```python
from build123d import *

# Parameters (mm, degrees)
SKETCH1_W               = 50.8
SKETCH1_H               = 304.8
BOSS_EXTRUDE1_DEPTH     = 3.175
CUT_EXTRUDE1_DEPTH      = 155.53478775
CUT_EXTRUDE1_DEPTH_BACK = 155.53478775
SKETCH2_R               = 3.175


with BuildPart() as part:
    # Sketch1 → Boss-Extrude1 (new, symmetric)
    with BuildSketch(Plane.XY):
        Rectangle(SKETCH1_W, SKETCH1_H)
    extrude(amount=BOSS_EXTRUDE1_DEPTH, both=True)

    # Sketch2 → Cut-Extrude1 (cut, two sides: drawn at the far end of the back side and taken through both)
    with BuildSketch(Plane.XY.offset(-CUT_EXTRUDE1_DEPTH_BACK)):
        with Locations((-12.7, 127)):
            Circle(SKETCH2_R)
        with Locations((12.7, 127)):
            Circle(SKETCH2_R)
        with Locations((12.7, 101.6)):
            Circle(SKETCH2_R)
        with Locations((12.7, 76.2)):
            Circle(SKETCH2_R)
        with Locations((12.7, 50.8)):
            Circle(SKETCH2_R)
        with Locations((12.7, 25.4)):
            Circle(SKETCH2_R)
        with Locations((12.7, 0)):
            Circle(SKETCH2_R)
        with Locations((12.7, -25.4)):
            Circle(SKETCH2_R)
        with Locations((12.7, -50.8)):
            Circle(SKETCH2_R)
        with Locations((12.7, -76.2)):
            Circle(SKETCH2_R)
        with Locations((12.7, -101.6)):
            Circle(SKETCH2_R)
        with Locations((-12.7, 101.6)):
            Circle(SKETCH2_R)
        with Locations((-12.7, 76.2)):
            Circle(SKETCH2_R)
        with Locations((-12.7, 50.8)):
            Circle(SKETCH2_R)
        with Locations((-12.7, 25.4)):
            Circle(SKETCH2_R)
        with Locations((-12.7, 0)):
            Circle(SKETCH2_R)
        with Locations((-12.7, -25.4)):
            Circle(SKETCH2_R)
        with Locations((-12.7, -50.8)):
            Circle(SKETCH2_R)
        with Locations((-12.7, -76.2)):
            Circle(SKETCH2_R)
        with Locations((-12.7, -101.6)):
            Circle(SKETCH2_R)
        with Locations((-12.7, -127)):
            Circle(SKETCH2_R)
        with Locations((12.7, -127)):
            Circle(SKETCH2_R)
    extrude(amount=CUT_EXTRUDE1_DEPTH + CUT_EXTRUDE1_DEPTH_BACK, mode=Mode.SUBTRACT)


solid = part.part
```
Geometry check sheet. Reference: the model listing, model coordinates, mm. Give positions to 0.01 mm unless a question says otherwise; leave off trailing zeros. Order: outer loops, then holes, each group sorted by start corner. A loop starts at its lowest first (then second) coordinate and runs counter-clockwise, first axis right, second up.
1. Release check for a two-part mould opening along X. For faces 1 (the face through (0, 152.4, 0)), 2 (the face through (-25.4, -2, 0)), 3 (the face through (12.29, -123.85, -0.04)) record: pulls with the +X half, pulls with the -X half, needs draft (parallel to the pull), parting line crosses it, or undercut.
2. Section check B-B, the plane z = 0.75. Give the number of separate pieces and of enclosed holes in the cut face, and give its area (3 significant figures).
3. Thickness scan on L1, parallel to X at y = 127, z = 1 (3 decimals); L2, parallel to X at y = 99, z = -1.75. Record the ranges inside material, lowest first.
4. Section check A-A, the plane y = 101.6. Enter the section's corners in (x, z) (3 decimals).
Values follow:
1. face 1: needs draft
1. face 2: pulls with the -X half
1. face 3: undercut
2. separate pieces: 1
2. enclosed holes: 22
2. area: 14,800 mm2
3. L1: x = -25.4 to -15.875, -9.525 to 9.525, 15.875 to 25.4
3. L2: x = -25.4 to -14.52, -10.88 to 10.88, 14.52 to 25.4
4. outline: (-25.4, -3.175) - (-15.875, -3.175) - (-15.875, 3.175) - (-25.4, 3.175) - close; (-9.525, -3.175) - (9.525, -3.175) - (9.525, 3.175) - (-9.525, 3.175) - close; (15.875, -3.175) - (25.4, -3.175) - (25.4, 3.175) - (15.875, 3.175) - close
